from build123d import *

# Parameters (mm, degrees)
MODEL_R             = 3.05
MODEL_R_2           = 2
BOSS_EXTRUDE1_DEPTH = 10


with BuildPart() as part:
    # Model → Boss-Extrude1 (new body)
    with BuildSketch(Plane.XY):
        with BuildLine():
            Line((-36, -25), (36, -25))
            ThreePointArc((36, -25), (38.828427125, -23.828427125), (40, -21))
            Line((40, -21), (40, 21))
            ThreePointArc((40, 21), (38.828427125, 23.828427125), (36, 25))
            Line((36, 25), (-36, 25))
            ThreePointArc((-36, 25), (-38.828427125, 23.828427125), (-40, 21))
            Line((-40, 21), (-40, -21))
            ThreePointArc((-40, -21), (-38.828427125, -23.828427125), (-36, -25))
        make_face()
        with Locations((-32, 17)):
            Circle(MODEL_R, mode=Mode.SUBTRACT)
        with Locations((32, -17)):
            Circle(MODEL_R, mode=Mode.SUBTRACT)
        with Locations((32, 17)):
            Circle(MODEL_R, mode=Mode.SUBTRACT)
        with Locations((-32, -17)):
            Circle(MODEL_R, mode=Mode.SUBTRACT)
        with Locations((-16, 17)):
            Circle(MODEL_R_2, mode=Mode.SUBTRACT)
        with Locations((16, 10)):
            Circle(MODEL_R_2, mode=Mode.SUBTRACT)
        with Locations((24, 10)):
            Circle(MODEL_R_2, mode=Mode.SUBTRACT)
        with Locations((-16, 3)):
            Circle(MODEL_R_2, mode=Mode.SUBTRACT)
        with Locations((-32, -4)):
            Circle(MODEL_R_2, mode=Mode.SUBTRACT)
        with Locations((32, 3)):
            Circle(MODEL_R_2, mode=Mode.SUBTRACT)
        with Locations((-16, -4)):
            Circle(MODEL_R_2, mode=Mode.SUBTRACT)
        with Locations((24, 3)):
            Circle(MODEL_R_2, mode=Mode.SUBTRACT)
        with Locations((16, 3)):
            Circle(MODEL_R_2, mode=Mode.SUBTRACT)
        with Locations((-16, 10)):
            Circle(MODEL_R_2, mode=Mode.SUBTRACT)
        with Locations((-8, 10)):
            Circle(MODEL_R_2, mode=Mode.SUBTRACT)
        with Locations((-32, 3)):
            Circle(MODEL_R_2, mode=Mode.SUBTRACT)
        with Locations((8, 10)):
            Circle(MODEL_R_2, mode=Mode.SUBTRACT)
        with Locations((16, 17)):
            Circle(MODEL_R_2, mode=Mode.SUBTRACT)
        with Locations((8, 17)):
            Circle(MODEL_R_2, mode=Mode.SUBTRACT)
        with Locations((0, 17)):
            Circle(MODEL_R_2, mode=Mode.SUBTRACT)
        with Locations((-8, 17)):
            Circle(MODEL_R_2, mode=Mode.SUBTRACT)
        with Locations((-16, -18)):
            Circle(MODEL_R_2, mode=Mode.SUBTRACT)
        with Locations((-8, -18)):
            Circle(MODEL_R_2, mode=Mode.SUBTRACT)
        with Locations((0, -18)):
            Circle(MODEL_R_2, mode=Mode.SUBTRACT)
        with Locations((8, -18)):
            Circle(MODEL_R_2, mode=Mode.SUBTRACT)
        with Locations((-24, -11)):
            Circle(MODEL_R_2, mode=Mode.SUBTRACT)
        with Locations((-24, -4)):
            Circle(MODEL_R_2, mode=Mode.SUBTRACT)
        with Locations((-24, 3)):
            Circle(MODEL_R_2, mode=Mode.SUBTRACT)
        with Locations((-24, 10)):
            Circle(MODEL_R_2, mode=Mode.SUBTRACT)
        with Locations((16, -18)):
            Circle(MODEL_R_2, mode=Mode.SUBTRACT)
        with Locations((-16, -11)):
            Circle(MODEL_R_2, mode=Mode.SUBTRACT)
        with Locations((24, -4)):
            Circle(MODEL_R_2, mode=Mode.SUBTRACT)
        with Locations((16, -4)):
            Circle(MODEL_R_2, mode=Mode.SUBTRACT)
        with Locations((32, -4)):
            Circle(MODEL_R_2, mode=Mode.SUBTRACT)
        with Locations((-8, -11)):
            Circle(MODEL_R_2, mode=Mode.SUBTRACT)
        with Locations((8, -11)):
            Circle(MODEL_R_2, mode=Mode.SUBTRACT)
        with Locations((16, -11)):
            Circle(MODEL_R_2, mode=Mode.SUBTRACT)
        with Locations((24, -11)):
            Circle(MODEL_R_2, mode=Mode.SUBTRACT)
        Polygon((6.380023856, -3.683453397), (6.379976144, 3.683536037), (-4.7712e-05, 7.366989435), (-6.380023856, 3.683453397), (-6.379976144, -3.683536037), (4.7712e-05, -7.366989435), align=None, mode=Mode.SUBTRACT)
    extrude(amount=BOSS_EXTRUDE1_DEPTH)


solid = part.part
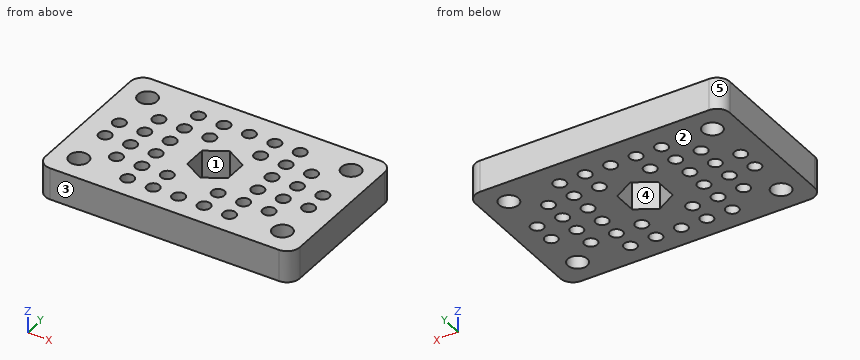
Read the model definition and answer for the solid it produces. Units are mm, in the model's axes. Face numbers are marked on the shaded views. A direction names the side the tool comes from. Give positions to 0.01 mm unless a question says otherwise; leave off trailing zeros. Loops run counter-clockwise (first coordinate to the right, second up) from the corner with the lowest first, then second, coordinate; pieces in that order, holes last. Notation, with made-up numbers: (39, 1) -> (44, 1) arc R24 ccw to (44, 27) -> close; hole circle Ø7 at (59, -6.75). An arc over 180 degrees is marked (long way). Use a Markdown table: item, result.
Q1. Section C-C, the plane x = 16 is taken. Determine the outline of the cut face in (y, z).
Solved:
| item | result |
|---|---|
| outline | (-25, 0) -> (-20, 0) -> (-20, 10) -> (-25, 10) -> close; (-16, 0) -> (-13, 0) -> (-13, 10) -> (-16, 10) -> close; (-9, 0) -> (-6, 0) -> (-6, 10) -> (-9, 10) -> close; (-2, 0) -> (1, 0) -> (1, 10) -> (-2, 10) -> close; (5, 0) -> (8, 0) -> (8, 10) -> (5, 10) -> close; (12, 0) -> (15, 0) -> (15, 10) -> (12, 10) -> close; (19, 0) -> (25, 0) -> (25, 10) -> (19, 10) -> close |
Q2. Section D-D, the plane y = -5 is taken. Count the separate pieces of the cut face and the enclosed holes in it, then the cut area to 3 significant figures.
Solved:
| item | result |
|---|---|
| separate pieces | 8 |
| enclosed holes | 0 |
| area | 510 mm^2 |
Q3. Determine the mould class of the marked faces 3, 4 and 5 for opening direction Y: pulls with the +Y half, pulls with the -Y half, needs draft (parallel to the pull), parting line crosses it, or undercut.
Solved:
| item | result |
|---|---|
| face 3 | pulls with the -Y half |
| face 4 | undercut |
| face 5 | pulls with the +Y half |
Q4. Find the intervals of material crossed by line 1 along Y through (x, z) = (-32, 7.75); line 2 along Y through (x, z) = (8, 3.25); line 3 along X through (y, z) = (-14.5, 8.5), in increasing order.
Solved:
| item | result |
|---|---|
| line 1 | y = -25 to -20.05, -13.95 to -6, -2 to 1, 5 to 13.95, 20.05 to 25 |
| line 2 | y = -25 to -20, -16 to -13, -9 to 8, 12 to 15, 19 to 25 |
| line 3 | x = -40 to -33.75, -30.25 to 30.25, 33.75 to 40 |
Q5. Section A-A, the plane y = -11 is taken. Determine the outline of the cut face in (x, z), then the cut area to 3 significant figures.
Solved:
| item | result |
|---|---|
| outline | (-40, 0) -> (-26, 0) -> (-26, 10) -> (-40, 10) -> close; (-22, 0) -> (-18, 0) -> (-18, 10) -> (-22, 10) -> close; (-14, 0) -> (-10, 0) -> (-10, 10) -> (-14, 10) -> close; (-6, 0) -> (6, 0) -> (6, 10) -> (-6, 10) -> close; (10, 0) -> (14, 0) -> (14, 10) -> (10, 10) -> close; (18, 0) -> (22, 0) -> (22, 10) -> (18, 10) -> close; (26, 0) -> (40, 0) -> (40, 10) -> (26, 10) -> close |
| area | 560 mm^2 |
Q6. A tool of negligible diameter and unlimited length cuts with its end or side. For the marked faces 1 and 2, from which of +Z, -Z, +X, -X, +Y, -Y can it reach the whole face along a straight path? Write none if from no direction.
Solved:
| item | result |
|---|---|
| face 1 | +Z, -Z |
| face 2 | -Z, +X, -X, +Y, -Y |
Q7. Section B-B, the plane x = 32 is taken. Determine the outline of the cut face in (y, z), then the cut area to 3 significant figures.
Solved:
| item | result |
|---|---|
| outline | (-25, 0) -> (-20.05, 0) -> (-20.05, 10) -> (-25, 10) -> close; (-13.95, 0) -> (-6, 0) -> (-6, 10) -> (-13.95, 10) -> close; (-2, 0) -> (1, 0) -> (1, 10) -> (-2, 10) -> close; (5, 0) -> (13.95, 0) -> (13.95, 10) -> (5, 10) -> close; (20.05, 0) -> (25, 0) -> (25, 10) -> (20.05, 10) -> close |
| area | 298 mm^2 |
